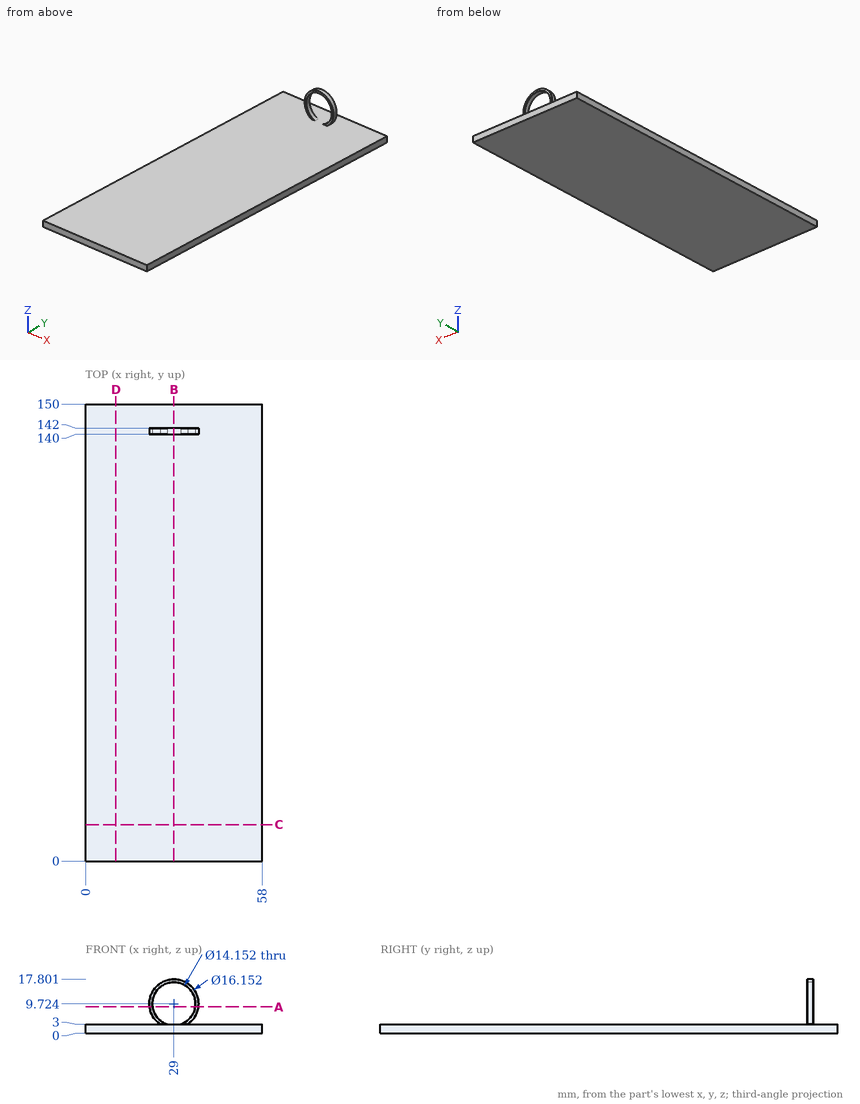
Part print with two shaded views. Sizes in mm from the minimum x, y, z corner. Coordinates: 2 decimals unless noted, no trailing zeros. Order: outer loops, then holes, each group sorted by start corner. A loop starts at its lowest first (then second) coordinate and runs counter-clockwise, first axis right, second up.
(1) Saw through at A-A, the plane z = 8.75. Write the cut outline in (x, y).
Solution:
outline: (20.98, 140) - (21.99, 140) - (21.99, 142) - (20.98, 142) - close; (36.01, 140) - (37.02, 140) - (37.02, 142) - (36.01, 142) - close
(2) Saw through at C-C, the plane y = 12. Write the cut outline in (x, z), and give its area (3 significant figures).
Solution:
outline: (0, 0) - (58, 0) - (58, 3) - (0, 3) - close
area: 174 mm2
(3) Pin check, flat tips, straight feed: pin 1 Ø10 at (x, z) = (11, 5) entering from -Y; pin 2 Ø2 at (x, z) = (21.5, 14) entering from -Y; pin 3 Ø8 at (x, y) = (50.5, 84.5) entering from +Z. Stop position of each tip, or through.
Solution:
pin 1: stops at y = 0
pin 2: stops at y = 140
pin 3: stops at z = 3
(4) Drill centre lines: L1, parallel to Z at x = 29, y = 140.75; L2, parallel to Y at x = 36.5, z = 10.25; L3, parallel to Z at x = 45.5, y = 121.5. Where is each one in solid material? Low to high.
Solution:
L1: z = 0 to 3, 16.8 to 17.8
L2: y = 140 to 142
L3: z = 0 to 3
(5) Saw through at B-B, the plane x = 29. Write the cut outline in (y, z), and give its area (3 significant figures).
Solution:
outline: (0, 0) - (150, 0) - (150, 3) - (0, 3) - close; (140, 16.8) - (142, 16.8) - (142, 17.8) - (140, 17.8) - close
area: 452 mm2
(6) Saw through at D-D, the plane x = 10. Write the cut outline in (y, z).
Solution:
outline: (0, 0) - (150, 0) - (150, 3) - (0, 3) - close
